Work out the finished part from the listing and answer in its coordinate system (mm). Face numbers are marked on the shaded views. A direction names the side the tool comes from. Round coordinates to 2 decimals unless told otherwise and drop trailing zeros. Loops run counter-clockwise (first coordinate to the right, second up) from the corner with the lowest first, then second, coordinate; pieces in that order, holes last.
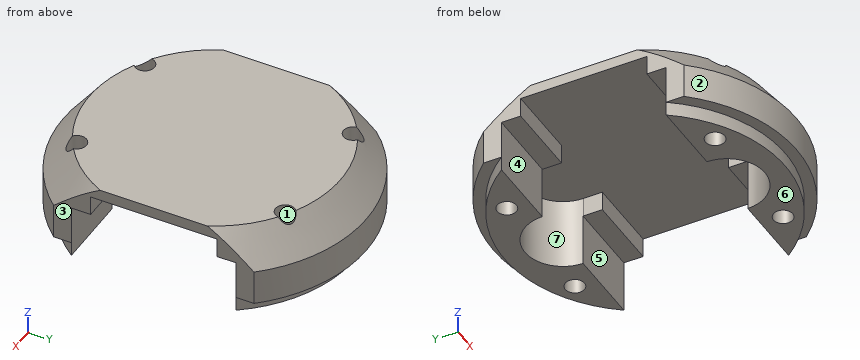
```python
from build123d import *

# Parameters (mm, degrees)
EXTRUDE1_DEPTH     = 2.25
EXTRUDE2_DEPTH     = 11
CHAMFER1_SIZE      = 4.1
CHAMFER1_SIZE2     = 5.440883769
SKETCH6_W          = 60
SKETCH6_H          = 26.1
CUT_EXTRUDE1_DEPTH = 8.4
SKETCH9_W          = 10
SKETCH9_H          = 40
CUT_EXTRUDE3_DEPTH = 37.143991781
SKETCH10_W         = 44
SKETCH10_H         = 20
CUT_EXTRUDE4_DEPTH = 3.1
CUT_EXTRUDE8_REACH = 34.796
SKETCH16_R         = 1.525
CUT_EXTRUDE9_DEPTH = 33.795769544


with BuildPart() as part:
    # Sketch1 → Extrude1 (new body)
    with BuildSketch(Plane.XY):
        with BuildLine():
            ThreePointArc((-22.224984725, -0.026057486), (0.013028745, -22.224996181), (22.225, 0))
            ThreePointArc((22.225, 0), (-0.013028745, 22.224996181), (-22.224984725, -0.026057486))
        make_face()
    extrude(amount=EXTRUDE1_DEPTH)

    # Sketch2 → Extrude2 (add)
    with BuildSketch(Plane.XY.offset(2.25)):
        with BuildLine():
            ThreePointArc((-23.999872331, -0.078282234), (0.113586787, -23.999731208), (23.999538151, 0.148891095))
            ThreePointArc((23.999538151, 0.148891095), (-0.113586787, 23.999731208), (-23.999872331, -0.078282234))
        make_face()
    extrude(amount=EXTRUDE2_DEPTH)

    # Chamfer1
    chamfer1_edges = [part.edges().sort_by_distance(p)[0] for p in [
        (-23.999538151, -0.148891095, 13.25),
    ]]
    chamfer1_side = [part.faces().sort_by_distance(p)[0] for p in [
        (0, 0, 13.25),
    ]]
    chamfer(chamfer1_edges, length=CHAMFER1_SIZE, length2=CHAMFER1_SIZE2, reference=chamfer1_side[0])

    # Sketch6 → Cut-Extrude1 (cut)
    with BuildSketch(Plane(origin=(0, 0, 0), x_dir=(-1, 0, 0), z_dir=(0, 0, -1))):
        Rectangle(SKETCH6_W, SKETCH6_H)
    extrude(amount=-CUT_EXTRUDE1_DEPTH, mode=Mode.SUBTRACT)

    # Sketch9 → Cut-Extrude3 (cut, through all)
    with BuildSketch(Plane(origin=(0, 0, 0), x_dir=(-1, 0, 0), z_dir=(0, 0, -1))):
        with Locations((-23, 0)):
            Rectangle(SKETCH9_W, SKETCH9_H)
        with Locations((23, 0)):
            Rectangle(SKETCH9_W, SKETCH9_H)
    extrude(amount=-CUT_EXTRUDE3_DEPTH, mode=Mode.SUBTRACT)

    # Sketch10 → Cut-Extrude4 (cut)
    with BuildSketch(Plane(origin=(0, 0, 8.4), x_dir=(-1, 0, 0), z_dir=(0, 0, -1))):
        Rectangle(SKETCH10_W, SKETCH10_H)
    extrude(amount=-CUT_EXTRUDE4_DEPTH, mode=Mode.SUBTRACT)

    # Cut-Extrude8: up to this face of the body (flat: up to its plane)
    cut_extrude8_end = Plane(part.part.faces().sort_by_distance((0, 0, 11.5))[0])
    # Sketch15 → Cut-Extrude8 (cut, up to the picked face)
    with BuildSketch(Plane(origin=(0, 0, 0), x_dir=(-1, 0, 0), z_dir=(0, 0, -1)), mode=Mode.PRIVATE) as cut_extrude8_sk1:
        with BuildLine():
            Line((6, -13), (6, 13))
            ThreePointArc((6, 13), (0, 19), (-6, 13))
            Line((-6, 13), (-6, -13))
            ThreePointArc((-6, -13), (0, -19), (6, -13))
        make_face()
    cut_extrude8_tool1 = split(extrude(cut_extrude8_sk1.sketch, amount=-CUT_EXTRUDE8_REACH, mode=Mode.PRIVATE), bisect_by=cut_extrude8_end, keep=Keep.BOTH, mode=Mode.PRIVATE)
    add(cut_extrude8_tool1.solids().sort_by(Axis((0, 0, 0), (0, 0, 1)))[0], mode=Mode.SUBTRACT)

    # Sketch16 → Cut-Extrude9 (cut, through all)
    with BuildSketch(Plane(origin=(0, 0, 0), x_dir=(-1, 0, 0), z_dir=(0, 0, -1))):
        with Locations((-10, -16.5)):
            Circle(SKETCH16_R)
        with Locations(Location((10, -16.5, 0), (0, 0, 9.857274388))):
            Circle(SKETCH16_R)
        with Locations((10, 16.5)):
            Circle(SKETCH16_R)
        with Locations(Location((-10, 16.5, 0), (0, 0, 52.579530574))):
            Circle(SKETCH16_R)
    extrude(amount=-CUT_EXTRUDE9_DEPTH, mode=Mode.SUBTRACT)


solid = part.part
```
1. Determine the mould class of the marked faces 1, 2, 3 and 4 for opening direction X: +X half, -X half, draft (parallel to the pull), parting line (faces both ways), or undercut.
Answer key:
face 1: undercut
face 2: parting line
face 3: +X half
face 4: draft
2. Which of the six approach directions +Z, -Z, +X, -X, +Y, -Y give full straight-line access (tool end or side, diameter ignored) to the marked faces 5, 6 and 7?
Answer key:
face 5: -Z, +X, -X
face 6: -Z, +X, -X, +Y, -Y
face 7: -Z
3. Find section B-B (z = 9.75). Write down the section's boundary in (x, y) (3 decimals).
Answer key:
outline: (-18, -13.562) arc R22.537 ccw to (18, -13.562) - (18, -10) - (6, -10) - (6, -13) arc R6 cw to (-6, -13) - (-6, -10) - (-18, -10) - close; (-18, 10) - (-6, 10) - (-6, 13) arc R6 cw to (6, 13) - (6, 10) - (18, 10) - (18, 13.562) arc R22.537 ccw to (-18, 13.562) - close; hole circle Ø3.05 at (-10, -16.5); hole circle Ø3.05 at (-10, 16.5); hole circle Ø3.05 at (10, -16.5); hole circle Ø3.05 at (10, 16.5)
4. Consider probe 1 along Y at (x, z) = (9, 6.5); probe 2 along X at (y, z) = (-16.5, 8) (3 decimals); probe 3 along X at (y, z) = (16.5, 8.25) (3 decimals). Determine where each line is inside the solid, lowest interval first.
Answer key:
probe 1: y = -22.25 to -17.65, -15.35 to -13.05, 13.05 to 15.35, 17.65 to 22.25
probe 2: x = -17.23 to -11.525, -8.475 to -4.873, 4.873 to 8.475, 11.525 to 17.23
probe 3: x = -16.968 to -11.525, -8.475 to -4.873, 4.873 to 8.475, 11.525 to 16.968
5. Find section A-A (z = 7.25). Give the number of separate pieces and of enclosed holes in the cut face, then the cut area to 3 significant figures.
Answer key:
separate pieces: 2
enclosed holes: 4
area: 468 mm2
6. Find section C-C (y = 2.5). Write down the section's boundary in (x, z), then the cut area to 3 significant figures.
Answer key:
outline: (-18, 11.5) - (18, 11.5) - (18, 13.25) - (-18, 13.25) - close
area: 63.0 mm2
7. Given pin 1 (3 mm diameter, centred on y = 11, z = 5.5, fed in from +X); pin 2 (4 mm diameter, centred on x = -14.5, z = 4.5, fed in from +Y); pin 3 (6 mm diameter, centred on x = -9.5, z = 9, fed in from +Y); pin 4 (0.9 mm diameter, centred on x = 11, z = 9.5, fed in from +Y), each flat-ended and moving along its own axis, determine where each tip first touches the part or whether it passes through.
Answer key:
pin 1: passes through
pin 2: stops at y = 20.49
pin 3: stops at y = 23.03
pin 4: stops at y = 20.34
